```python
from build123d import *

# Parameters (mm, degrees)
F0_R          = 15
F1_DEPTH      = 10
F2_R          = 2
F3_R          = 5
F4_DEPTH      = 5
F5_R          = 5
F6_DEPTH      = 5
F7_R          = 6
F8_DEPTH      = 15.001
F8_DEPTH_BACK = 15.001


with BuildPart() as f1:
    # F0 (on Top) → F1 (new body, symmetric)
    with BuildSketch(Plane.XY):
        Circle(F0_R)
    extrude(amount=F1_DEPTH, both=True)

    # F2
    f2_edges = [f1.edges().sort_by_distance(p)[0] for p in [
        (-15, 0, 10),
        (-15, 0, -10),
    ]]
    fillet(f2_edges, radius=F2_R)

    # F3 (on face) → F4 (join)
    with BuildSketch(Plane.XY.offset(10)):
        Circle(F3_R)
    extrude(amount=F4_DEPTH)

    # F5 (on face) → F6 (join)
    with BuildSketch(Plane(origin=(0, 0, -10), x_dir=(1, 0, 0), z_dir=(0, 0, -1))):
        Circle(F5_R)
    extrude(amount=F6_DEPTH)

    # F7 (on Front) → F8 (cut, two sides)
    with BuildSketch(Plane.XZ) as f8_sk:
        Circle(F7_R)
    extrude(amount=F8_DEPTH, mode=Mode.SUBTRACT)
    extrude(f8_sk.sketch, amount=-F8_DEPTH_BACK, mode=Mode.SUBTRACT)


solid = f1.part
```
Input: part model. Units: mm. Frame: model coordinates. A direction names the side the tool comes from. Give positions to 0.01 mm unless a question says otherwise; leave off trailing zeros. Order: outer loops, then holes, each group sorted by start corner. A loop starts at its lowest first (then second) coordinate and runs counter-clockwise, first axis right, second up. Notation, with made-up numbers: (-16.75, 72) - (-0.75, 72) arc R20 cw to (-0.75, 94) - close; hole circle Ø11 at (52.5, -25). An arc over 180 degrees is marked (long way). One line per item, written item: value.
1. Cut plane B-B, the plane z = 3.5. Output: boundary loops of the cut face in (x, y).
Determined:
outline: (-4.87, -14.19) - (-4.87, 14.19) arc R15 ccw to start; (4.87, -14.19) arc R15 ccw to (4.87, 14.19) - close
2. Cut plane C-C, the plane z = 0. Output: boundary loops of the cut face in (x, y).
Determined:
outline: (-6, -13.75) - (-6, 13.75) arc R15 ccw to start; (6, -13.75) arc R15 ccw to (6, 13.75) - close
3. Line query: probe 1 along Z at (x, y) = (0, 10.5); probe 2 along Z at (x, y) = (-1.5, -8); probe 3 along X at (y, z) = (8.5, -4.25). Output: solid intervals per line, ascending.
Determined:
probe 1: -10 to -6, 6 to 10
probe 2: -10 to -5.81, 5.81 to 10
probe 3: -12.36 to -4.24, 4.24 to 12.36
4. Pin query (flat end, axial travel): pin 1 Ø2 at (x, y) = (-2, -11) entering from +Z; pin 2 Ø10 at (y, z) = (11, -7.5) entering from -X; pin 3 Ø11 at (x, z) = (0, 0) entering from -Y; pin 4 Ø5 at (x, y) = (-9, 0) entering from -Z. Return the tip coordinate at first contact, or that it passes through.
Determined:
pin 1: z = 10
pin 2: x = -13.75
pin 3: through
pin 4: z = -10
5. Reachability of faces 1 (the face through (-1.08, -4.88, 12.46)), 2 (the face through (0, 0, 15)), 3 (the face through (-1.08, 4.88, -12.46)) from +Z, -Z, +X, -X, +Y, -Y: full face, straight path, thin tool, end or side. Return the list, or none.
Determined:
face 1: +Z
face 2: +Z, +X, -X, +Y, -Y
face 3: -Z
6. Cut plane A-A, the plane x = 0. Output: boundary loops of the cut face in (y, z).
Determined:
outline: (-15, -8) arc R2 ccw to (-13, -10) - (-5, -10) - (-5, -15) - (5, -15) - (5, -10) - (13, -10) arc R2 ccw to (15, -8) - (15, -6) - (-15, -6) - close; (-15, 6) - (15, 6) - (15, 8) arc R2 ccw to (13, 10) - (5, 10) - (5, 15) - (-5, 15) - (-5, 10) - (-13, 10) arc R2 ccw to (-15, 8) - close
